The drawing under review shows one solid part. Ordinate dimensions are in mm from its lowest x, y, z. Give positions to 0.01 mm unless a question says otherwise; leave off trailing zeros. Order: outer loops, then holes, each group sorted by start corner. A loop starts at its lowest first (then second) coordinate and runs counter-clockwise, first axis right, second up. Notation, with made-up numbers: (63, 27) -> (91, 27) arc R15 ccw to (91, 31) -> close; hole circle Ø6 at (-28.75, 15). An arc over 180 degrees is marked (long way). Return JSON: item names as keys, results as strings. Group by question number.
1) To check wall thickness, follow line 1 along Y through (x, z) = (36.5, 7.5); line 2 along X through (y, z) = (25, 12.5); line 3 along X through (y, z) = (37.5, 13.25). State the ranges of each line that lie inside material, in increasing order.
2) Add section B-B (z = 10). Give the boundary of the cut face in (x, y).
3) Add section A-A (x = 3.5). Give the boundary of the cut face in (y, z).
4) The part is to be moulded in two halves that separate along X. For the marked faces 1, 2 and 3, say which applies: released by +X, released by -X, zero draft, split by the parting line, or undercut.
5) Insertion check: P1, Ø2, axis at x = 36.5, y = 20, coming from the -Z side. The pin has a flat end and moves straight along its axis. Give the tip position at first contact, or say it passes through.
6) Add section C-C (y = 20). Give the boundary of the cut face in (x, z).
7) Add section D-D (y = 32). Give the boundary of the cut face in (x, z).
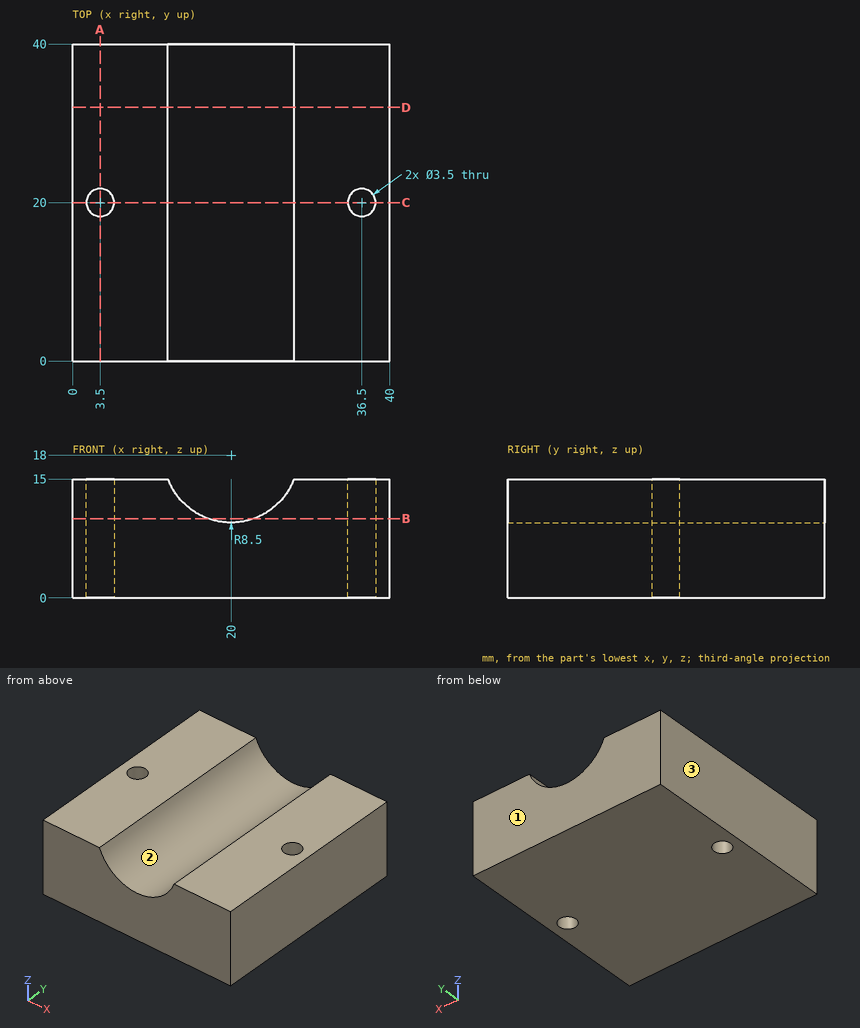
Evaluation:
{
 "1": {"line 1": "0 to 18.25, 21.75 to 40", "line 2": "0 to 13.52, 26.48 to 40", "line 3": "0 to 12.95, 27.05 to 40"},
 "2": {"outline": "(0, 0) -> (17.13, 0) -> (17.13, 40) -> (0, 40) -> close; (22.87, 0) -> (40, 0) -> (40, 40) -> (22.87, 40) -> close; hole circle Ø3.5 at (3.5, 20); hole circle Ø3.5 at (36.5, 20)"},
 "3": {"outline": "(0, 0) -> (18.25, 0) -> (18.25, 15) -> (0, 15) -> close; (21.75, 0) -> (40, 0) -> (40, 15) -> (21.75, 15) -> close"},
 "4": {"face 1": "zero draft", "face 2": "undercut", "face 3": "released by -X"},
 "5": {"P1": "through"},
 "6": {"outline": "(0, 0) -> (1.75, 0) -> (1.75, 15) -> (0, 15) -> close; (5.25, 0) -> (34.75, 0) -> (34.75, 15) -> (27.95, 15) arc R8.5 cw to (12.05, 15) -> (5.25, 15) -> close; (38.25, 0) -> (40, 0) -> (40, 15) -> (38.25, 15) -> close"},
 "7": {"outline": "(0, 0) -> (40, 0) -> (40, 15) -> (27.95, 15) arc R8.5 cw to (12.05, 15) -> (0, 15) -> close"}
}
